Can you work these out from the model? Positions are in its coordinate system, mm. Give positions to 0.01 mm unless a question says otherwise; leave off trailing zeros. Write each loop counter-clockwise with the first axis right and the second up, starting at its lowest first coordinate (ties: lowest second). Pieces come first, ordered by that corner, then holes.
from build123d import *

# Parameters (mm, degrees)
F0_R     = 139.7
F0_R_2   = 85.09
F1_DEPTH = 25.4
F3_D     = 22.225


with BuildPart() as f1:
    # F0 (on Front) → F1 (new body)
    with BuildSketch(Plane.XZ):
        Circle(F0_R)
        Circle(F0_R_2, mode=Mode.SUBTRACT)
    extrude(amount=F1_DEPTH)

    # F3 (through all)
    with Locations(Plane.XZ.offset(25.4)):
        with Locations((-85.312433, 85.312433), (0, 120.65), (85.312433, 85.312433), (120.65, 0), (85.312433, -85.312433), (0, -120.65), (-85.312433, -85.312433), (-120.65, 0)):
            Hole(F3_D / 2)


solid = f1.part
(1) If we mould it in two halves opening along Z, with no side actions, what happens to faces 1 (the face through (-110.86, -12.52, -85.01)), 2 (the face through (-109.55, -12.52, 0.49)), 3 (the face through (60, -25.4, 64))? For each: +Z half, -Z half, draft (parallel to the pull), parting line (faces both ways), or undercut.
Returned:
face 1: parting line
face 2: undercut
face 3: draft
(2) Imagine slicing it at C-C, the plane y = -18. Give the number of separate pieces and of enclosed holes in the cut face, plus the area to 3 significant figures.
Returned:
separate pieces: 1
enclosed holes: 9
area: 35,500 mm2
(3) Imagine slicing it at B-B, the plane z = 120.65. Write out the boundary of the cut face in (x, y).
Returned:
outline: (-70.42, -25.4) - (-11.11, -25.4) - (-11.11, 0) - (-70.42, 0) - close; (11.11, -25.4) - (70.42, -25.4) - (70.42, 0) - (11.11, 0) - close
(4) Will these pins go through, and if not, where does the flat tip stop? P1, Ø20, axis at x = 0, z = 120.65, coming from the +Y side; P2, Ø1.5, axis at x = 17.5, y = -9.5, coming from the +Z side; P3, Ø2, axis at x = -39.5, y = -22, coming from the -Z side; P4, Ø4, axis at x = 68.5, y = -16, coming from the +Z side.
Returned:
P1: passes through
P2: stops at z = 138.69
P3: stops at z = -134.29
P4: stops at z = 122.86
(5) Imagine slicing it at A-A, the plane x = 66.5. Write out the boundary of the cut face in (y, z).
Returned:
outline: (-25.4, -122.86) - (0, -122.86) - (0, -53.09) - (-25.4, -53.09) - close; (-25.4, 53.09) - (0, 53.09) - (0, 122.86) - (-25.4, 122.86) - close
(6) Imagine slicing it at D-D, the plane x = -89. Write out the boundary of the cut face in (y, z), plus the area to 3 significant figures.
Returned:
outline: (-25.4, -107.68) - (0, -107.68) - (0, -95.8) - (-25.4, -95.8) - close; (-25.4, -74.83) - (0, -74.83) - (0, 74.83) - (-25.4, 74.83) - close; (-25.4, 95.8) - (0, 95.8) - (0, 107.68) - (-25.4, 107.68) - close
area: 4,410 mm2
(7) If I drill on L1, parallel to Z at x = 0, y = -10.25; L2, parallel to Z at x = 6, y = -2; L3, parallel to X at y = -19.5, z = 9, over which ranges is the centre line in solid material (lowest first)?
Returned:
L1: z = -139.7 to -131.76, -109.54 to -85.09, 85.09 to 109.54, 131.76 to 139.7
L2: z = -139.57 to -130, -111.3 to -84.88, 84.88 to 111.3, 130 to 139.57
L3: x = -139.41 to -127.17, -114.13 to -84.61, 84.61 to 114.13, 127.17 to 139.41
